The listing builds one solid part. Answer for the finished solid, in the listing's coordinates (mm). A direction names the side the tool comes from. Round coordinates to 2 decimals unless told otherwise and drop trailing zeros. Loops run counter-clockwise (first coordinate to the right, second up) from the corner with the lowest first, then second, coordinate; pieces in that order, holes last. Notation, with made-up numbers: M 17,39 L 44,39 A26 cw 44,60 Z; hole C 24.5,-16.5 d4. An arc over 180 degrees is marked long. Put each result on its own line as item: value. Start each with the question number.
(1) Straight lines are drawn through the part: line 1 (Y direction, x = 55, z = 2); line 2 (Y direction, x = 0, z = 6); line 3 (Z direction, x = -9.5, y = -39). For each, find the intervals that lie inside material, in ascending order.
(2) Section C-C, the plane z = 11.5 is taken. Determine the outline of the cut face in (x, y), then the cut area to 3 significant figures.
(3) Flat-ended cylindrical pins translate along their axes: P1, Ø10, axis at x = 38.5, z = 21.5, coming from the +Y side; P2, Ø6, axis at y = -19.5, z = 29.5, coming from the +X side; P3, Ø5, axis at x = -55, y = 50, coming from the -Z side; P4, Ø3, axis at x = 17, z = 43, coming from the -Y side. Find the tip coordinate at first contact, or state that the pin passes through.
(4) Determine the mould class of faces 4 (the face through (-9.678, -43.584, 19.854)), 5 (the face through (58, -54, 2)), 6 (the face through (-1, 55, 1)) for opening direction Y: released by +Y, released by -Y, zero draft, split by the parting line, or undercut.
(5) Which of the six approach directions +Z, -Z, +X, -X, +Y, -Y give full straight-line access (tool end or side, diameter ignored) to faces 1 (the face through (-20, -15.33, 36.11)), 2 (the face through (-58, -54, 2)), 3 (the face through (-10.3, -46.37, 8.38))?
```python
from build123d import *

# Parameters (mm, degrees)
SKETCH_W        = 120
SKETCH_H        = 110
SKETCH_R        = 1.5
SKETCH_R_2      = 47.5
PAD_DEPTH       = 3
SKETCH001_R     = 50.5
SKETCH001_R_2   = 47.5
PAD001_DEPTH    = 17
SKETCH008_R     = 50.5
SKETCH008_R_2   = 22
PAD005_DEPTH    = 4
SKETCH004_R     = 30
SKETCH004_R_2   = 25.2
PAD004_DEPTH    = 2
SKETCH009_R     = 25.2
SKETCH009_R_2   = 22
PAD006_DEPTH    = 24
CHAMFER_SIZE    = 2
CHAMFER001_SIZE = 1.5
FILLET_R        = 5
FILLET001_R     = 5
FILLET002_R     = 5


with BuildPart() as part:
    # Sketch → Pad (new body)
    with BuildSketch(Plane.XY):
        Rectangle(SKETCH_W, SKETCH_H)
        with Locations((-55, 50)):
            Circle(SKETCH_R, mode=Mode.SUBTRACT)
        with Locations((-55, -50)):
            Circle(SKETCH_R, mode=Mode.SUBTRACT)
        with Locations((55, 50)):
            Circle(SKETCH_R, mode=Mode.SUBTRACT)
        with Locations((55, -50)):
            Circle(SKETCH_R, mode=Mode.SUBTRACT)
        Circle(SKETCH_R_2, mode=Mode.SUBTRACT)
    extrude(amount=PAD_DEPTH)

    # Sketch001 (on Face11 of Pad) → Pad001 (join)
    with BuildSketch(Plane.XY.offset(3)):
        Circle(SKETCH001_R)
        Circle(SKETCH001_R_2, mode=Mode.SUBTRACT)
    extrude(amount=PAD001_DEPTH)

    # Sketch008 (on Face14 of Pad001) → Pad005 (join)
    with BuildSketch(Plane.XY.offset(20)):
        Circle(SKETCH008_R)
        Circle(SKETCH008_R_2, mode=Mode.SUBTRACT)
    extrude(amount=PAD005_DEPTH)

    # Sketch004 → Pad004 (join)
    with BuildSketch(Plane.XY.offset(24)):
        Circle(SKETCH004_R)
        Circle(SKETCH004_R_2, mode=Mode.SUBTRACT)
    extrude(amount=PAD004_DEPTH)

    # Sketch009 (on Face16 of Pad004) → Pad006 (join)
    with BuildSketch(Plane.XY.offset(24)):
        Circle(SKETCH009_R)
        Circle(SKETCH009_R_2, mode=Mode.SUBTRACT)
    extrude(amount=PAD006_DEPTH)

    # Sketch005 → Revolution (revolve)
    with BuildSketch(Plane.XZ):
        Polygon((47.5, 20), (47.5, 17), (44.5, 20), align=None)
    revolve(axis=Axis((0, 0, 0), (0, 0, 1)))

    # Sketch006 → Revolution001 (revolve)
    with BuildSketch(Plane.XZ):
        Polygon((50.5, 6), (50.5, 3), (53.5, 3), align=None)
    revolve(axis=Axis((0, 0, 0), (0, 0, 1)))

    # Chamfer
    chamfer_edges = [part.edges().sort_by_distance(p)[0] for p in [
        (-50.5, 0, 24),
    ]]
    chamfer(chamfer_edges, length=CHAMFER_SIZE)

    # Chamfer001
    chamfer001_edges = [part.edges().sort_by_distance(p)[0] for p in [
        (-25.2, 0, 48),
    ]]
    chamfer(chamfer001_edges, length=CHAMFER001_SIZE)

    # Fillet
    fillet_edges = [part.edges().sort_by_distance(p)[0] for p in [
        (60, 55, 1.5),
        (60, -55, 1.5),
    ]]
    fillet(fillet_edges, radius=FILLET_R)

    # Fillet001
    fillet001_edges = [part.edges().sort_by_distance(p)[0] for p in [
        (-60, -55, 1.5),
    ]]
    fillet(fillet001_edges, radius=FILLET001_R)

    # Fillet002
    fillet002_edges = [part.edges().sort_by_distance(p)[0] for p in [
        (-60, 55, 1.5),
    ]]
    fillet(fillet002_edges, radius=FILLET002_R)


solid = part.part
```
Recorded:
1. line 1: y = -55 to -51.5, -48.5 to 48.5, 51.5 to 55
1. line 2: y = -50.5 to -47.5, 47.5 to 50.5
1. line 3: z = 20 to 24
2. outline: C 0,0 d101; hole C 0,0 d95
2. area: 924 mm²
3. P1: stops at y = 37.79
3. P2: stops at x = 19.05
3. P3: stops at z = 0
3. P4: stops at y = -19.87
4. face 4: undercut
4. face 5: released by -Y
4. face 6: released by +Y
5. face 1: +Z
5. face 2: +Z, -Z, -X, -Y
5. face 3: -Z
